from build123d import *

# Parameters (mm, degrees)
SKETCH3_W           = 457.2
SKETCH3_H           = 609.6
SKETCH3_R           = 3.175
BOSS_EXTRUDE1_DEPTH = 3.175
FILLET1_R           = 6.35


with BuildPart() as part:
    # Sketch3 → Boss-Extrude1 (new body)
    with BuildSketch(Plane(origin=(0, 0, 0), x_dir=(0, 0.3173046564050865, -0.9483236552062013), z_dir=(0, -0.9483236552062012, -0.3173046564050864))):
        Rectangle(SKETCH3_W, SKETCH3_H)
        with Locations((203.2, -270.933333333)):
            Circle(SKETCH3_R, mode=Mode.SUBTRACT)
        with Locations((-203.2, -270.933333333)):
            Circle(SKETCH3_R, mode=Mode.SUBTRACT)
        with Locations((-203.2, 270.933333333)):
            Circle(SKETCH3_R, mode=Mode.SUBTRACT)
        with Locations((203.2, 270.933333333)):
            Circle(SKETCH3_R, mode=Mode.SUBTRACT)
    extrude(amount=-BOSS_EXTRUDE1_DEPTH)

    # Fillet1
    fillet1_edges = [part.edges().sort_by_distance(p)[0] for p in [
        (-304.8, 74.041308257, -216.283066438),
        (-304.8, -71.030380652, 217.290508722),
        (304.8, -71.030380652, 217.290508722),
        (304.8, 74.041308257, -216.283066438),
    ]]
    fillet(fillet1_edges, radius=FILLET1_R)


solid = part.part
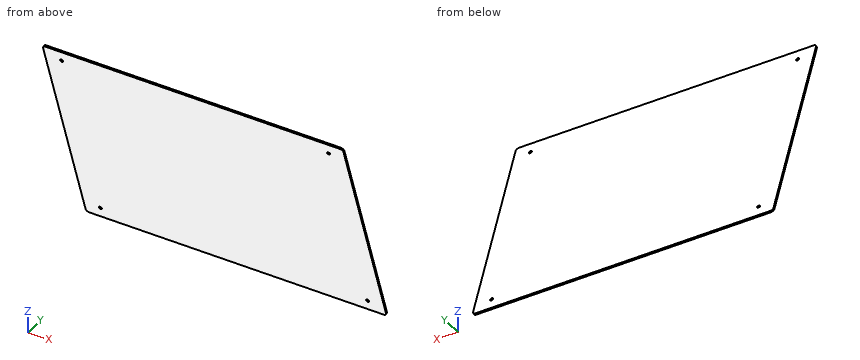
For this review, take the finished solid that the model builds, in its own axes (mm). Give positions to 0.01 mm unless a question says otherwise; leave off trailing zeros. Loops run counter-clockwise (first coordinate to the right, second up) from the corner with the lowest first, then second, coordinate; pieces in that order, holes last. Notation, with made-up numbers: (-27, 7.25) -> (-3, 7.25) arc R16 cw to (-3, 14.25) -> close; hole circle Ø1 at (-6.75, -1.5). An arc over 180 degrees is marked (long way). One line per question, with ' | ' between items.
1) To check wall thickness, follow probe 1 along Y at (x, z) = (217, 2.5); probe 2 along Y at (x, z) = (-121, 48.5). State the ranges of each line that lie inside material, in increasing order.
Resolved:
probe 1: y = -0.84 to 2.51 | probe 2: y = -16.23 to -12.88
2) We need section A-A (x = 32). Write out the cut boundary in (y, z).
Resolved:
outline: (-72.54, 216.79) -> (72.54, -216.79) -> (75.55, -215.78) -> (-69.52, 217.79) -> close
3) Insertion check: pin 1 Ø10 at (x, z) = (128, 123.5) entering from -Y; pin 2 Ø1.5 at (x, z) = (-81.5, -10) entering from +Y; pin 3 Ø2 at (x, z) = (-124, -86) entering from -Y. Each pin has a flat end and moves straight along its axis. Give the tip position at first contact, or say it passes through.
Resolved:
pin 1: stops at y = -43 | pin 2: stops at y = 6.94 | pin 3: stops at y = 28.44
4) We need section B-B (y = -28.5). Write out the cut boundary in (x, z).
Resolved:
outline: (-304.8, 85.18) -> (304.8, 85.18) -> (304.8, 95.18) -> (-304.8, 95.18) -> close
